CAD build for the part. Positions are in the model's coordinates, mm. Face numbers are marked on the shaded views. Round coordinates to 2 decimals unless told otherwise and drop trailing zeros. Order: outer loops, then holes, each group sorted by start corner. A loop starts at its lowest first (then second) coordinate and runs counter-clockwise, first axis right, second up. Notation, with made-up numbers: M 70.25,34 L 96.25,34 A10 cw 96.25,43 Z; hole C -31.5,-4.5 d10. An arc over 180 degrees is marked long. Put each result on its own line as item: value.
```python
from build123d import *

# Parameters (mm, degrees)
SKETCH1_R           = 20
BOSS_EXTRUDE1_DEPTH = 5
SKETCH3_R           = 1.5
CUT_EXTRUDE1_DEPTH  = 5


with BuildPart() as part:
    # Sketch1 → Boss-Extrude1 (new body)
    with BuildSketch(Plane.XY):
        Circle(SKETCH1_R)
    extrude(amount=BOSS_EXTRUDE1_DEPTH)

    # Sketch3 → Cut-Extrude1 (cut)
    with BuildSketch(Plane.XY.offset(5)):
        with Locations((0, 20)):
            Circle(SKETCH3_R)
        with Locations((5.176380902, 19.318516526)):
            Circle(SKETCH3_R)
        with Locations((10, 17.320508076)):
            Circle(SKETCH3_R)
        with Locations((14.142135624, 14.142135624)):
            Circle(SKETCH3_R)
        with Locations((17.320508076, 10)):
            Circle(SKETCH3_R)
        with Locations((19.318516526, 5.176380902)):
            Circle(SKETCH3_R)
        with Locations((20, 0)):
            Circle(SKETCH3_R)
        with Locations((19.318516526, -5.176380902)):
            Circle(SKETCH3_R)
        with Locations((17.320508076, -10)):
            Circle(SKETCH3_R)
        with Locations((14.142135624, -14.142135624)):
            Circle(SKETCH3_R)
        with Locations((10, -17.320508076)):
            Circle(SKETCH3_R)
        with Locations((5.176380902, -19.318516526)):
            Circle(SKETCH3_R)
        with Locations((0, -20)):
            Circle(SKETCH3_R)
        with Locations((-5.176380902, -19.318516526)):
            Circle(SKETCH3_R)
        with Locations((-10, -17.320508076)):
            Circle(SKETCH3_R)
        with Locations((-14.142135624, -14.142135624)):
            Circle(SKETCH3_R)
        with Locations((-17.320508076, -10)):
            Circle(SKETCH3_R)
        with Locations((-19.318516526, -5.176380902)):
            Circle(SKETCH3_R)
        with Locations((-20, 0)):
            Circle(SKETCH3_R)
        with Locations((-19.318516526, 5.176380902)):
            Circle(SKETCH3_R)
        with Locations((-17.320508076, 10)):
            Circle(SKETCH3_R)
        with Locations((-14.142135624, 14.142135624)):
            Circle(SKETCH3_R)
        with Locations((-10, 17.320508076)):
            Circle(SKETCH3_R)
        with Locations((-5.176380902, 19.318516526)):
            Circle(SKETCH3_R)
    extrude(amount=-CUT_EXTRUDE1_DEPTH, mode=Mode.SUBTRACT)


solid = part.part
```
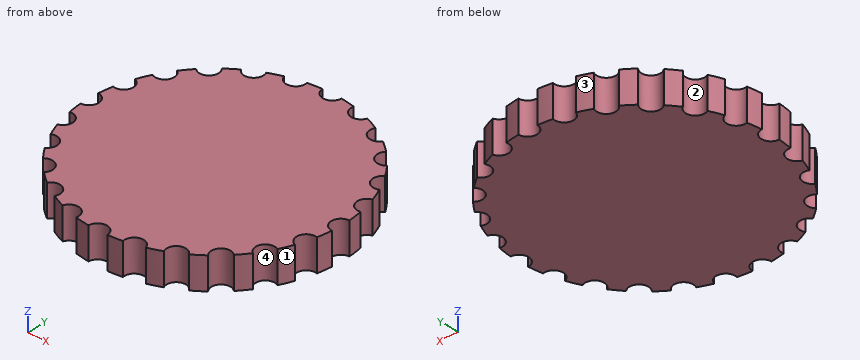
Item 1: Probe line 1 along Y through (x, z) = (18, 1.2); line 2 along X through (y, z) = (-15.5, 2.4); line 3 along X through (y, z) = (-12, 1.2). List the from-to ranges inside material, lowest first. Write a range as [from, to].
Answers below:
line 1: [-8.66, -5.89], [-4.46, 4.46], [5.89, 8.66]
line 2: [-12.64, 12.64]
line 3: [-16, 16]
Item 2: Band-saw the part on A-A on x = -10. Give the cut face in (y, z).
Answers below:
outline: M -15.82,0 L 15.82,0 L 15.82,5 L -15.82,5 Z
Item 3: Mould opens along Y. For the marked faces 1, 2, 3 and 4 say: pulls with the +Y half, pulls with the -Y half, needs draft (parallel to the pull), parting line crosses it, or undercut.
Answers below:
face 1: pulls with the -Y half
face 2: undercut
face 3: pulls with the +Y half
face 4: undercut
